from build123d import *

# Parameters (mm, degrees)
F1_DEPTH = 14.5
F2_START = 5
F0_W     = 1.5
F0_H     = 2
F2_DEPTH = 4.5
F3_SIZE  = 0.5
F4_SIZE2 = 1.5
F4_SIZE  = 2
F5_R     = 0.4


with BuildPart() as f1:
    # F0 (on Top) → F1 (new body)
    with BuildSketch(Plane.XY):
        Polygon((0, 2), (0, 0), (10, 0), (10, 8.5), (10, 10.5), (7.9, 10.5), (7.9, 2), align=None)
    extrude(amount=F1_DEPTH)

    # F0 (on Top) → F2 (join)
    with BuildSketch(Plane.XY.offset(F2_START)):
        with Locations((10.75, 9.5)):
            Rectangle(F0_W, F0_H)
    extrude(amount=F2_DEPTH)

    # F3
    f3_edges = [f1.edges().sort_by_distance(p)[0] for p in [
        (10, 0, 7.25),
    ]]
    chamfer(f3_edges, length=F3_SIZE)

    # F4
    f4_edges = [f1.edges().sort_by_distance(p)[0] for p in [
        (11.5, 10.5, 7.25),
    ]]
    f4_side = f1.faces().sort_by_distance((9.276613, 10.5, 7.25))[0]
    chamfer(f4_edges, length=F4_SIZE, length2=F4_SIZE2, reference=f4_side)

    # F5
    f5_edges = [f1.edges().sort_by_distance(p)[0] for p in [
        (11.5, 8.5, 7.25),
    ]]
    fillet(f5_edges, radius=F5_R)


solid = f1.part
Could you check a few things on this model? Use its own coordinates, in mm. A direction names the side the tool comes from. Coordinates: 2 decimals unless noted, no trailing zeros. Loops run counter-clockwise (first coordinate to the right, second up) from the corner with the lowest first, then second, coordinate; pieces in that order, holes last.
1. Imagine slicing it at C-C (x = 3). Please give me the cut outline in (y, z), and give its area (3 significant figures).
2. Imagine slicing it at A-A (z = 8.75). Please give me the cut outline in (x, y), and give its area (3 significant figures).
3. Imagine slicing it at D-D (z = 2.75). Please give me the cut outline in (x, y) (3 decimals).
4. Imagine slicing it at B-B (y = 2.5). Please give me the cut outline in (x, z), and give its area (4 significant figures).
5. For P1, Ø1.5, axis at y = 4.5, z = 11, coming from the +X side; P2, Ø4, axis at x = 2, z = 10.5, coming from the +Y side; P3, Ø0.9, axis at x = 10.5, z = 7, coming from the -Y side, each with a flat end and sliding along its axis, tell me the tip position at first contact or that it passes through.
6. I need wall thicknesses on L1, parallel to Y at x = 6.5, z = 11.5; L2, parallel to X at y = 4.25, z = 11; L3, parallel to X at y = 1, z = 4.25. Which ranges of each line are inside material? Lowest first, please.
7. For faces 1 (the face through (0, 1, 7)), 2 (the face through (11, 9, 5)), 3 (the face through (11, 9, 9.5)), 4 (the face through (4, 2, 7)), 5 (the face through (10.5, 8.5, 7.2)), which set-ups out of +Z, -Z, +X, -X, +Y, -Y let a thin tool reach every point of the face, with its end or its side?
Computed values:
1. outline: (0, 0) - (2, 0) - (2, 14.5) - (0, 14.5) - close
1. area: 29.0 mm2
2. outline: (0, 0) - (9.5, 0) - (10, 0.5) - (10, 8.5) - (11.1, 8.5) arc R0.4 ccw to (11.5, 8.9) - (11.5, 9) - (9.5, 10.5) - (7.9, 10.5) - (7.9, 2) - (0, 2) - close
2. area: 39.2 mm2
3. outline: (0, 0) - (9.5, 0) - (10, 0.5) - (10, 10.125) - (9.5, 10.5) - (7.9, 10.5) - (7.9, 2) - (0, 2) - close
4. outline: (7.9, 0) - (10, 0) - (10, 14.5) - (7.9, 14.5) - close
4. area: 30.45 mm2
5. P1: stops at x = 10
5. P2: stops at y = 2
5. P3: stops at y = 8.5
6. L1: y = 0 to 2
6. L2: x = 7.9 to 10
6. L3: x = 0 to 10
7. face 1: +Z, -Z, -X, +Y, -Y
7. face 2: -Z, +X, +Y, -Y
7. face 3: +Z, +X, +Y, -Y
7. face 4: +Z, -Z, -X, +Y
7. face 5: +Z, -Z, +X, -Y
